Geometry check sheet. Reference: drawing and pictorial views, mm from the part's lowest x, y, z. A direction names the side the tool comes from. Give positions to 0.01 mm unless a question says otherwise; leave off trailing zeros. Loops run counter-clockwise (first coordinate to the right, second up) from the corner with the lowest first, then second, coordinate; pieces in that order, holes last. Notation, with made-up numbers: M 40,85.5 L 87,85.5 A14 ccw 87,91.5 Z; hole C -40,44 d9. An arc over 180 degrees is marked long. Use CSV: the item, a comma, the result in double quotes.
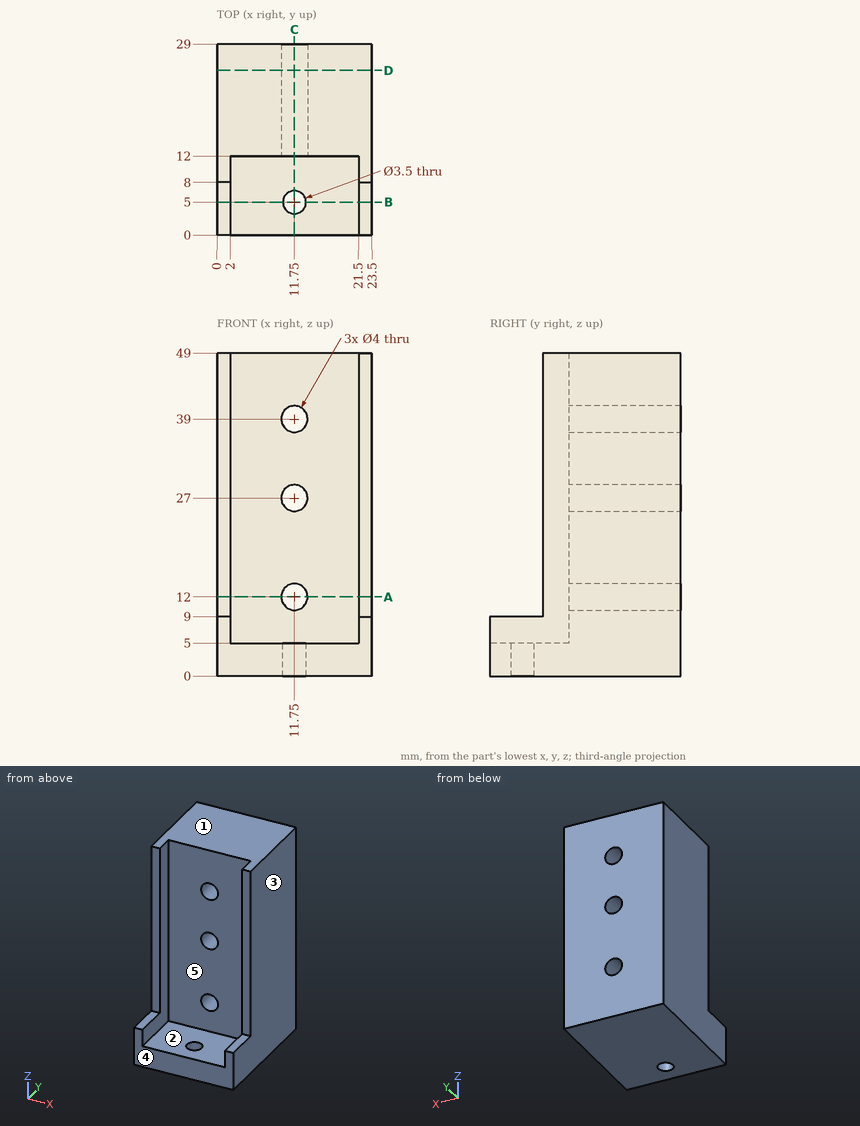
(1) Scan lines: L1, parallel to Y at x = 11.75, z = 1.7; L2, parallel to Z at x = 13.5, y = 24; L3, parallel to X at y = 19.75, z = 12. Record each from-to range of solid material in increasing order. Write a range as from..to.
Calculated:
L1,"y = 0..3.25, 6.75..29"
L2,"z = 0..11.03, 12.97..26.03, 27.97..38.03, 39.97..49"
L3,"x = 0..9.75, 13.75..23.5"
(2) Section check C-C on x = 11.75. Record the cut outline in (y, z), plus the area to 4 significant figures.
Calculated:
outline,"M 0,0 L 3.25,0 L 3.25,5 L 0,5 Z; M 6.75,0 L 29,0 L 29,10 L 12,10 L 12,5 L 6.75,5 Z; M 12,14 L 29,14 L 29,25 L 12,25 Z; M 12,29 L 29,29 L 29,37 L 12,37 Z; M 12,41 L 29,41 L 29,49 L 12,49 Z"
area,"671.5 mm²"
(3) Depth check by flat-ended pin: pin 1 Ø1.6 at (x, z) = (1.5, 37) entering from -Y; pin 2 Ø3 at (x, z) = (16, 30.5) entering from -Y; pin 3 Ø1.6 at (x, y) = (1, 4) entering from +Z; pin 4 Ø1 at (x, y) = (9.5, 15.5) entering from -Z. Enter the tip coordinate at first touch or a pass-through.
Calculated:
pin 1,"stops at y = 8"
pin 2,"stops at y = 12"
pin 3,"stops at z = 9"
pin 4,"stops at z = 0"
(4) Section check D-D on y = 25. Record the cut outline in (x, z), plus the area to 3 significant figures.
Calculated:
outline,"M 0,0 L 23.5,0 L 23.5,49 L 0,49 Z; hole C 11.75,12 d4; hole C 11.75,27 d4; hole C 11.75,39 d4"
area,"1,110 mm²"
(5) Tool access check on the marked faces 4 and 5. Record the directions out of +Z, -Z, +X, -X, +Y, -Y that give a thin tool (end or side, any length) a straight path to the whole face; none if there is none.
Calculated:
face 4,"+Z, -Z, +X, -X, -Y"
face 5,"+Z, -Y"
(6) Mould release check, pull along X, two halves, no side actions. Record for the marked faces 1, 2 and 3: released by +X, released by -X, zero draft, split by the parting line, or undercut.
Calculated:
face 1,"zero draft"
face 2,"undercut"
face 3,"released by +X"
(7) Section check A-A on z = 12. Record the cut outline in (x, y), plus the area to 4 significant figures.
Calculated:
outline,"M 0,8 L 2,8 L 2,12 L 9.75,12 L 9.75,29 L 0,29 Z; M 13.75,12 L 21.5,12 L 21.5,8 L 23.5,8 L 23.5,29 L 13.75,29 Z"
area,"347.5 mm²"
(8) Section check B-B on y = 5. Record the cut outline in (x, z), plus the area to 3 significant figures.
Calculated:
outline,"M 0,0 L 10,0 L 10,5 L 2,5 L 2,9 L 0,9 Z; M 13.5,0 L 23.5,0 L 23.5,9 L 21.5,9 L 21.5,5 L 13.5,5 Z"
area,"116 mm²"
